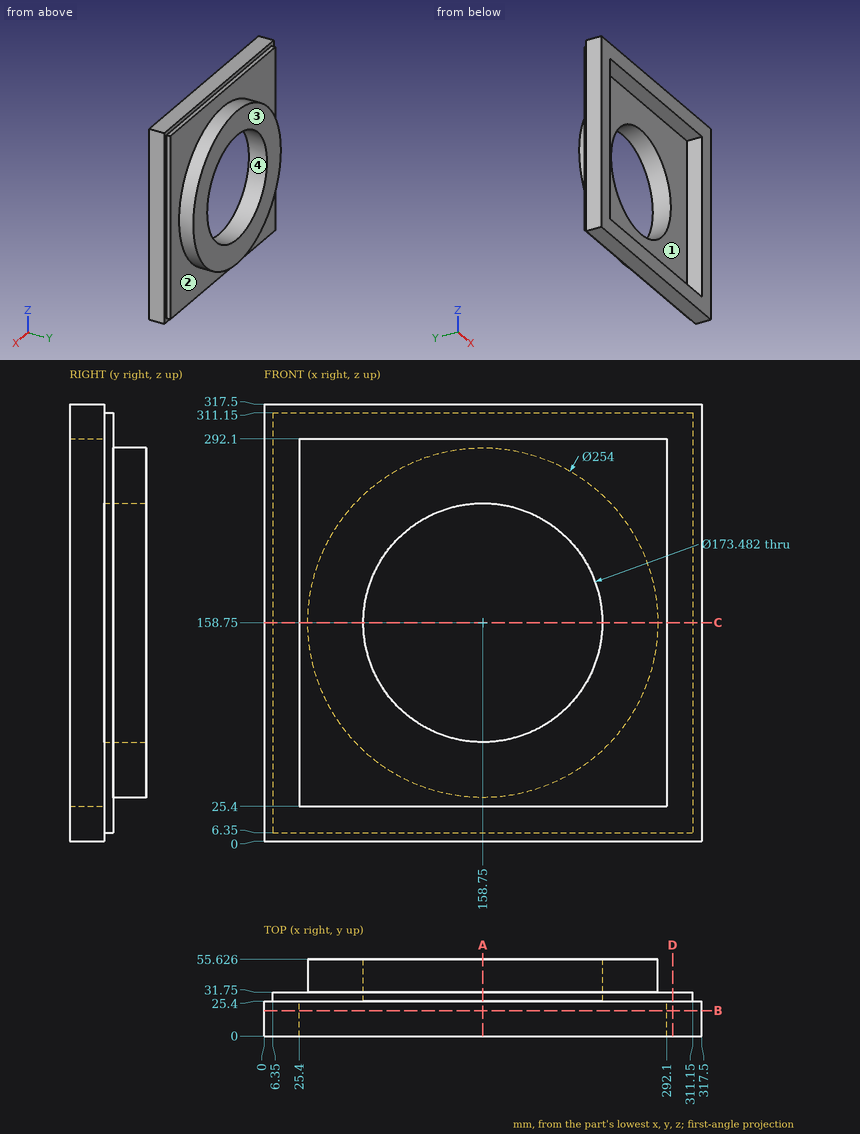
Check sheet for the drawn part. Datum: minimum x, y, z corner. Units: mm. A direction names the side the tool comes from. Coordinates: 2 decimals unless noted, no trailing zeros. Loops run counter-clockwise (first coordinate to the right, second up) from the corner with the lowest first, then second, coordinate; pieces in that order, holes last. Notation, with made-up numbers: (84.5, 55) -> (134.5, 55) arc R18 ccw to (134.5, 79) -> close; hole circle Ø3 at (-29, 43.5). An arc over 180 degrees is marked (long way). Answer as CSV lines item,"result".
1) Cross-section at A-A, the plane x = 158.75. Record the cut outline in (y, z), then the cut area to 3 significant figures.
Found:
outline,"(0, 0) -> (25.4, 0) -> (25.4, 6.35) -> (31.75, 6.35) -> (31.75, 31.75) -> (55.63, 31.75) -> (55.63, 72.01) -> (25.4, 72.01) -> (25.4, 25.4) -> (0, 25.4) -> close; (0, 292.1) -> (25.4, 292.1) -> (25.4, 245.49) -> (55.63, 245.49) -> (55.63, 285.75) -> (31.75, 285.75) -> (31.75, 311.15) -> (25.4, 311.15) -> (25.4, 317.5) -> (0, 317.5) -> close"
area,"4,050 mm2"
2) Depth check by flat-ended pin: pin 1 (6 mm diameter, centred on y = 48, z = 169.5, fed in from +X); pin 2 (4 mm diameter, centred on x = 34, z = 275, fed in from -Y); pin 3 (1.9 mm diameter, centred on y = 30, z = 95.5, fed in from -X). Enter the tip coordinate at first touch or a pass-through.
Found:
pin 1,"stops at x = 285.51"
pin 2,"stops at y = 25.4"
pin 3,"stops at x = 6.35"
3) Cross-section at D-D, the plane x = 296.5. Record the cut outline in (y, z).
Found:
outline,"(0, 0) -> (25.4, 0) -> (25.4, 6.35) -> (31.75, 6.35) -> (31.75, 311.15) -> (25.4, 311.15) -> (25.4, 317.5) -> (0, 317.5) -> close"
4) Cross-section at C-C, the plane z = 158.75. Record the cut outline in (x, y).
Found:
outline,"(0, 0) -> (25.4, 0) -> (25.4, 25.4) -> (72.01, 25.4) -> (72.01, 55.63) -> (31.75, 55.63) -> (31.75, 31.75) -> (6.35, 31.75) -> (6.35, 25.4) -> (0, 25.4) -> close; (245.49, 25.4) -> (292.1, 25.4) -> (292.1, 0) -> (317.5, 0) -> (317.5, 25.4) -> (311.15, 25.4) -> (311.15, 31.75) -> (285.75, 31.75) -> (285.75, 55.63) -> (245.49, 55.63) -> close"
5) Release check for a two-part mould opening along Z. For the marked faces 3 and 4 record: +Z half, -Z half, draft (parallel to the pull), parting line (faces both ways), or undercut.
Found:
face 3,"draft"
face 4,"undercut"
6) Tool access check on the marked faces 1 and 2. Record the directions out of +Z, -Z, +X, -X, +Y, -Y that give a thin tool (end or side, any length) a straight path to the whole face; none if there is none.
Found:
face 1,"-Y"
face 2,"+Y"
7) Thickness scan on L1, parallel to Z at x = 288, y = 13; L2, parallel to Z at x = 158.75, y = 42.5. Record the ranges inside material, lowest first. Write a range as from..to.
Found:
L1,"z = 0..25.4, 292.1..317.5"
L2,"z = 31.75..72.01, 245.49..285.75"
8) Cross-section at B-B, the plane y = 18.5. Record the cut outline in (x, z).
Found:
outline,"(0, 0) -> (317.5, 0) -> (317.5, 317.5) -> (0, 317.5) -> close; hole (25.4, 25.4) -> (292.1, 25.4) -> (292.1, 292.1) -> (25.4, 292.1) -> close"
